Verification items for the finished model (mm, model axes). A direction names the side the tool comes from. Coordinates: 2 decimals unless noted, no trailing zeros. Order: outer loops, then holes, each group sorted by start corner. A loop starts at its lowest first (then second) coordinate and runs counter-clockwise, first axis right, second up. Notation, with made-up numbers: (72.5, 52.25) - (84.5, 52.25) arc R13 ccw to (84.5, 71.25) - close; hole circle Ø1 at (11.5, 55). An arc over 180 degrees is marked (long way). Answer as CSV lines item,"result". Start each with the question number.
1. Section check B-B (y = 6.5). Record the cut outline in (x, z), and give its area (3 significant figures).
2. Material ranges on L1, parallel to Z at x = 300.5, y = -0.5; L2, parallel to X at y = 2.5, z = 7.5, recorded low to high. Write a range as [from, to].
3. Section check A-A (x = 490.5). Record the cut outline in (y, z), and give its area (3 significant figures).
4. Mould release check, pull along X, two halves, no side actions. Record for faces 1 (the flat face through (598, 0, 0)), 2 (the flat face through (295, 10, 0)), 3 (the flat face through (294, 0, 4)): pulls with the +X half, pulls with the -X half, needs draft (parallel to the pull), parting line crosses it, or undercut.
5. Set-up check for faces 4 (the flat face through (295, -10, 0)), 5 (the flat face through (301, 0, -6)): record each of +Z, -Z, +X, -X, +Y, -Y from which the full face is reachable in a straight line by a thin tool's end or side.
from build123d import *

# Parameters (mm, degrees)
F0_W     = 20
F0_H     = 60
F1_DEPTH = 598
F3_DEPTH = 25


with BuildPart() as f1:
    # F0 (on Right) → F1 (new body)
    with BuildSketch(Plane.YZ):
        Rectangle(F0_W, F0_H)
    extrude(amount=F1_DEPTH)

    # F2 (on face) → F3 (cut)
    with BuildSketch(Plane.XZ.offset(10)):
        with BuildLine():
            Line((535, 12), (60, 12))
            ThreePointArc((60, 12), (56, 8), (60, 4))
            Line((60, 4), (535, 4))
            ThreePointArc((535, 4), (539, 8), (535, 12))
        make_face()
        with BuildLine():
            Line((535, -6), (60, -6))
            ThreePointArc((60, -6), (56, -10), (60, -14))
            Line((60, -14), (535, -14))
            ThreePointArc((535, -14), (539, -10), (535, -6))
        make_face()
    extrude(amount=-F3_DEPTH, mode=Mode.SUBTRACT)


solid = f1.part
Evaluation:
1,outline,"(0, -30) - (598, -30) - (598, 30) - (0, 30) - close; hole (60, -14) - (535, -14) arc R4 ccw to (535, -6) - (60, -6) arc R4 ccw to start; hole (60, 4) - (535, 4) arc R4 ccw to (535, 12) - (60, 12) arc R4 ccw to start"
1,area,"28,200 mm²"
2,L1,"z = [-30, -14], [-6, 4], [12, 30]"
2,L2,"x = [0, 56.03], [538.97, 598]"
3,outline,"(-10, -30) - (10, -30) - (10, -14) - (-10, -14) - close; (-10, -6) - (10, -6) - (10, 4) - (-10, 4) - close; (-10, 12) - (10, 12) - (10, 30) - (-10, 30) - close"
3,area,"880 mm²"
4,face 1,"pulls with the +X half"
4,face 2,"needs draft"
4,face 3,"undercut"
5,face 4,"+Z, -Z, +X, -X, -Y"
5,face 5,"+Y, -Y"
